```python
from build123d import *

# Parameters (mm, degrees)
SKETCH1_R               = 7.5
BOSS_EXTRUDE1_DEPTH     = 7
SKETCH2_R               = 8.5
BOSS_EXTRUDE2_DEPTH     = 3
SKETCH3_R               = 7.5
BOSS_EXTRUDE3_DEPTH     = 7
CUT_EXTRUDE3_DEPTH      = 8
CUT_EXTRUDE3_DEPTH_BACK = 11
SKETCH7_R               = 10.5
SKETCH7_R_2             = 8.5
BOSS_EXTRUDE4_DEPTH     = 3


with BuildPart() as part:
    # Sketch1 → Boss-Extrude1 (new body)
    with BuildSketch(Plane.XY):
        Circle(SKETCH1_R)
    extrude(amount=BOSS_EXTRUDE1_DEPTH)

    # Sketch2 → Boss-Extrude2 (add)
    with BuildSketch(Plane.XY.offset(7)):
        with Locations((0, 1)):
            Circle(SKETCH2_R)
    extrude(amount=BOSS_EXTRUDE2_DEPTH)

    # Sketch3 → Boss-Extrude3 (add)
    with BuildSketch(Plane.XY.offset(10)):
        with Locations((0, 2)):
            Circle(SKETCH3_R)
    extrude(amount=BOSS_EXTRUDE3_DEPTH)

    # Sketch6 → Cut-Extrude3 (cut, two sides)
    with BuildSketch(Plane.XY.offset(10)) as cut_extrude3_sk:
        with BuildLine():
            Line((-2.449489743, 3.5), (2.449489743, 3.5))
            ThreePointArc((2.449489743, 3.5), (3.5, 1), (2.449489743, -1.5))
            Line((2.449489743, -1.5), (-2.449489743, -1.5))
            ThreePointArc((-2.449489743, -1.5), (-3.5, 1), (-2.449489743, 3.5))
        make_face()
    extrude(amount=CUT_EXTRUDE3_DEPTH, mode=Mode.SUBTRACT)
    extrude(cut_extrude3_sk.sketch, amount=-CUT_EXTRUDE3_DEPTH_BACK, mode=Mode.SUBTRACT)

    # Sketch7 → Boss-Extrude4 (add)
    with BuildSketch(Plane.XY.offset(10)):
        with Locations((0, 1)):
            Circle(SKETCH7_R)
        with Locations((0, 1)):
            Circle(SKETCH7_R_2, mode=Mode.SUBTRACT)
    extrude(amount=-BOSS_EXTRUDE4_DEPTH)


solid = part.part
```
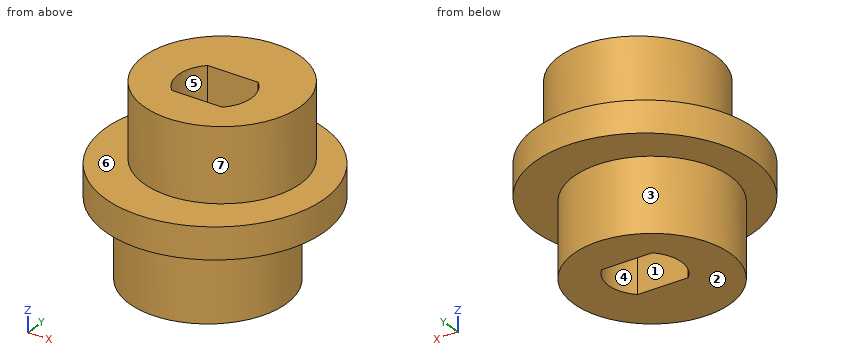
The listing builds one solid part. Answer for the finished solid, in the listing's coordinates (mm). Face numbers are marked on the shaded views. A direction names the side the tool comes from. Round coordinates to 2 decimals unless told otherwise and drop trailing zeros. Order: outer loops, then holes, each group sorted by start corner. A loop starts at its lowest first (then second) coordinate and runs counter-clockwise, first axis right, second up. Notation, with made-up numbers: (49, 40) - (87, 40) arc R21 cw to (87, 54) - close; hole circle Ø9 at (32, 84.25). An arc over 180 degrees is marked (long way). Put each result on its own line as item: value. Start each with the question number.
(1) Find section A-A (x = 2.75). Give the vertices of the cut face in (y, z), plus the area to 3 significant figures.
(2) Find section C-C (y = 0). Give the vertices of the cut face in (x, z).
(3) Find section B-B (z = 2). Give the vertices of the cut face in (x, y).
(4) Determine the mould class of the marked faces 4, 5, 6 and 7 for opening direction X: released by +X, released by -X, zero draft, split by the parting line, or undercut.
(5) Find section D-D (y = -3.5). Give the vertices of the cut face in (x, z), plus the area to 3 significant figures.
(6) Given P1, Ø4, axis at y = 0, z = 4.5, coming from the -X side; P2, Ø3, axis at x = -2, y = 1.5, coming from the +Z side; P3, Ø4, axis at y = 6.5, z = 5.5, coming from the -X side; P4, Ø1, axis at y = -5, z = 11.5, coming from the -X side, each flat-ended and moving along its own axis, determine where each tip first touches the part or whether it passes through.
(7) For the marked faces 1, 2 and 3, determine the directions among +Z, -Z, +X, -X, +Y, -Y from which every point of the face is accessible in a straight line to the end or side of a thin tool.
(8) Straight lines are drawn through the part: probe 1 along Y at (x, z) = (0, 10.5); probe 2 along Y at (x, z) = (-0.75, 9); probe 3 along X at (y, z) = (1.75, 9). For each, find the intervals that lie inside material, in ascending order. Write a range as from..to.
Reply:
1. outline: (-9.13, 7) - (-6.98, 7) - (-6.98, 0) - (-1.17, 0) - (-1.17, 17) - (-4.98, 17) - (-4.98, 10) - (-9.13, 10) - close; (3.17, 0) - (6.98, 0) - (6.98, 7) - (11.13, 7) - (11.13, 10) - (8.98, 10) - (8.98, 17) - (3.17, 17) - close
1. area: 183 mm^2
2. outline: (-10.45, 7) - (-7.5, 7) - (-7.5, 0) - (-3.35, 0) - (-3.35, 17) - (-7.23, 17) - (-7.23, 10) - (-10.45, 10) - close; (3.35, 0) - (7.5, 0) - (7.5, 7) - (10.45, 7) - (10.45, 10) - (7.23, 10) - (7.23, 17) - (3.35, 17) - close
3. outline: circle Ø15 at (0, 0); hole (-2.45, -1.5) - (2.45, -1.5) arc R3.5 ccw to (2.45, 3.5) - (-2.45, 3.5) arc R3.5 ccw to start
4. face 4: undercut
4. face 5: undercut
4. face 6: zero draft
4. face 7: split by the parting line
5. outline: (-9.49, 7) - (-6.63, 7) - (-6.63, 0) - (6.63, 0) - (6.63, 7) - (9.49, 7) - (9.49, 10) - (5.1, 10) - (5.1, 17) - (-5.1, 17) - (-5.1, 10) - (-9.49, 10) - close
5. area: 221 mm^2
6. P1: x = -7.5
6. P2: z = 17
6. P3: x = -9.63
6. P4: x = -3.74
7. face 1: +Z, -Z
7. face 2: -Z, +X, -X, +Y, -Y
7. face 3: -Z
8. probe 1: -5.5..-1.5, 3.5..9.5
8. probe 2: -9.47..-1.5, 3.5..11.47
8. probe 3: -10.47..-3.42, 3.42..10.47
